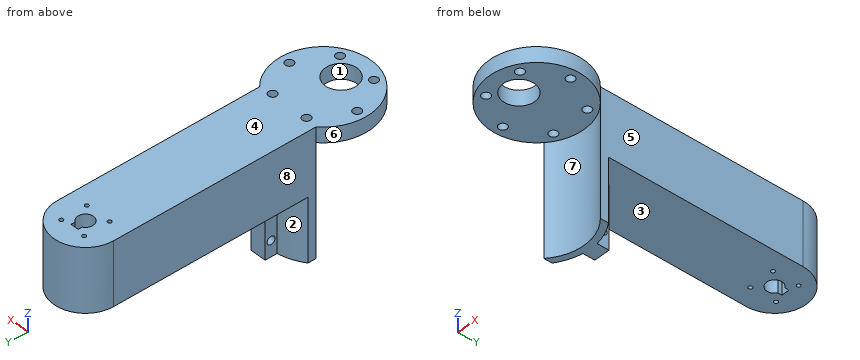
from build123d import *

# Parameters (mm, degrees)
SKETCH1_R           = 3.175
SKETCH1_R_2         = 0.762
BOSS_EXTRUDE1_DEPTH = 25.4
SKETCH2_R           = 19.05
SKETCH2_R_2         = 3.175
BOSS_EXTRUDE2_DEPTH = 25.4
SKETCH3_R           = 1.651
CUT_EXTRUDE1_DEPTH  = 25.4
SKETCH5_R           = 6.35
CUT_EXTRUDE2_DEPTH  = 25.4
SKETCH6_W           = 3.175
SKETCH6_H           = 1.5875
CUT_EXTRUDE3_DEPTH  = 25.4
SKETCH2_2_R         = 3.175
CUT_EXTRUDE6_DEPTH  = 25.4
SKETCH8_R           = 1.651
SKETCH8_R_2         = 6.35
CUT_EXTRUDE4_DEPTH  = 19.3
BOSS_EXTRUDE3_DEPTH = 25.4
SKETCH10_W          = 6.35
SKETCH10_H          = 4.7625
BOSS_EXTRUDE4_DEPTH = 25.4
SKETCH11_R          = 1.5875
CUT_EXTRUDE5_DEPTH  = 23.225


with BuildPart() as part:
    # Sketch1 → Boss-Extrude1 (new body)
    with BuildSketch(Plane.XY):
        with BuildLine():
            Line((12.7, 50.8), (12.7, -50.8))
            ThreePointArc((12.7, -50.8), (0, -63.5), (-12.7, -50.8))
            Line((-12.7, -50.8), (-12.7, 50.8))
            ThreePointArc((-12.7, 50.8), (0, 63.5), (12.7, 50.8))
        make_face()
        with Locations((0, 50.8)):
            Circle(SKETCH1_R, mode=Mode.SUBTRACT)
        with Locations((-5.118745989, 55.918745989)):
            Circle(SKETCH1_R_2, mode=Mode.SUBTRACT)
        with Locations((5.118745989, 55.918745989)):
            Circle(SKETCH1_R_2, mode=Mode.SUBTRACT)
        with Locations((5.118745989, 45.681254011)):
            Circle(SKETCH1_R_2, mode=Mode.SUBTRACT)
        with Locations((-5.118745989, 45.681254011)):
            Circle(SKETCH1_R_2, mode=Mode.SUBTRACT)
    extrude(amount=BOSS_EXTRUDE1_DEPTH)

    # Sketch2 → Boss-Extrude2 (add)
    with BuildSketch(Plane(origin=(0, 0, 0), x_dir=(-1, 0, 0), z_dir=(0, 0, -1))):
        with Locations((0, -44.45)):
            Circle(SKETCH2_R)
        with Locations((0, 50.8)):
            Circle(SKETCH2_R_2)
    extrude(amount=-BOSS_EXTRUDE2_DEPTH)

    # Sketch3 → Cut-Extrude1 (cut)
    with BuildSketch(Plane.XY.offset(25.4)):
        with Locations((-7.62, -30.959275928)):
            Circle(SKETCH3_R)
        with Locations((7.62, -30.959275928)):
            Circle(SKETCH3_R)
        with Locations((-15.24, -44.45)):
            Circle(SKETCH3_R)
        with Locations((-7.62, -57.940724072)):
            Circle(SKETCH3_R)
        with Locations((7.62, -57.940724072)):
            Circle(SKETCH3_R)
        with Locations((15.24, -44.45)):
            Circle(SKETCH3_R)
    extrude(amount=-CUT_EXTRUDE1_DEPTH, mode=Mode.SUBTRACT)

    # Sketch5 → Cut-Extrude2 (cut)
    with BuildSketch(Plane.XY.offset(25.4)):
        with Locations((0, -51.562)):
            Circle(SKETCH5_R)
    extrude(amount=-CUT_EXTRUDE2_DEPTH, mode=Mode.SUBTRACT)

    # Sketch6 → Cut-Extrude3 (cut)
    with BuildSketch(Plane(origin=(0, 0, 0), x_dir=(-1, 0, 0), z_dir=(0, 0, -1))):
        with Locations((0, 54.343380657)):
            Rectangle(SKETCH6_W, SKETCH6_H)
    extrude(amount=-CUT_EXTRUDE3_DEPTH, mode=Mode.SUBTRACT)

    # Sketch2<2> → Cut-Extrude6 (cut)
    with BuildSketch(Plane(origin=(0, 0, 0), x_dir=(-1, 0, 0), z_dir=(0, 0, -1))):
        with Locations((0, 50.8)):
            Circle(SKETCH2_2_R)
    extrude(amount=-CUT_EXTRUDE6_DEPTH, mode=Mode.SUBTRACT)

    # Sketch8 → Cut-Extrude4 (cut)
    with BuildSketch(Plane(origin=(0, 0, 0), x_dir=(-1, 0, 0), z_dir=(0, 0, -1))):
        with BuildLine():
            ThreePointArc((-12.7, -30.250968343), (-7.777129933, -61.840191201), (19.05, -44.45))
            ThreePointArc((19.05, -44.45), (17.390191201, -36.672870067), (12.7, -30.250968343))
            ThreePointArc((12.7, -30.250968343), (0, -25.4), (-12.7, -30.250968343))
        make_face()
        with Locations((-7.62, -57.940724072)):
            Circle(SKETCH8_R, mode=Mode.SUBTRACT)
        with Locations((7.62, -57.940724072)):
            Circle(SKETCH8_R, mode=Mode.SUBTRACT)
        with Locations((0, -51.562)):
            Circle(SKETCH8_R_2, mode=Mode.SUBTRACT)
        with Locations((-15.24, -44.45)):
            Circle(SKETCH8_R, mode=Mode.SUBTRACT)
        with Locations((-7.62, -30.959275928)):
            Circle(SKETCH8_R, mode=Mode.SUBTRACT)
        with Locations((15.24, -44.45)):
            Circle(SKETCH8_R, mode=Mode.SUBTRACT)
        with Locations((7.62, -30.959275928)):
            Circle(SKETCH8_R, mode=Mode.SUBTRACT)
        with Locations((7.62, -30.959275928)):
            Circle(SKETCH8_R)
        with Locations((-7.62, -30.959275928)):
            Circle(SKETCH8_R)
        with Locations((-15.24, -44.45)):
            Circle(SKETCH8_R)
        with Locations((-7.62, -57.940724072)):
            Circle(SKETCH8_R)
        with Locations((0, -51.562)):
            Circle(SKETCH8_R_2)
        with Locations((7.62, -57.940724072)):
            Circle(SKETCH8_R)
        with Locations((15.24, -44.45)):
            Circle(SKETCH8_R)
    extrude(amount=-CUT_EXTRUDE4_DEPTH, mode=Mode.SUBTRACT)

    # Sketch9 → Boss-Extrude3 (add)
    with BuildSketch(Plane(origin=(0, 0, 0), x_dir=(-1, 0, 0), z_dir=(0, 0, -1))):
        with BuildLine():
            Line((-12.7, -30.250968343), (-12.7, -26.990386602))
            ThreePointArc((-12.7, -26.990386602), (0, -22.86), (12.7, -26.990386602))
            Line((12.7, -26.990386602), (12.7, -30.250968343))
            ThreePointArc((12.7, -30.250968343), (0, -25.4), (-12.7, -30.250968343))
        make_face()
    extrude(amount=BOSS_EXTRUDE3_DEPTH)

    # Sketch10 → Boss-Extrude4 (add)
    with BuildSketch(Plane(origin=(0, 0, 0), x_dir=(-1, 0, 0), z_dir=(0, 0, -1))):
        with Locations((0, -20.713481915)):
            Rectangle(SKETCH10_W, SKETCH10_H)
    extrude(amount=BOSS_EXTRUDE4_DEPTH)

    # Sketch11 → Cut-Extrude5 (cut, through all)
    with BuildSketch(Plane(origin=(3.175, 0, 0), x_dir=(0, 0, -1), z_dir=(1, 0, 0))):
        with Locations((6.35, -20.713481915)):
            Circle(SKETCH11_R)
        with Locations((19.05, -20.713481915)):
            Circle(SKETCH11_R)
    extrude(amount=-CUT_EXTRUDE5_DEPTH, mode=Mode.SUBTRACT)


solid = part.part
The model under review builds one solid part; all positions refer to its coordinate system, in mm. Face numbers are marked on the shaded views. A direction names the side the tool comes from. Coordinates: 2 decimals unless noted, no trailing zeros. Order: outer loops, then holes, each group sorted by start corner. A loop starts at its lowest first (then second) coordinate and runs counter-clockwise, first axis right, second up. Notation, with made-up numbers: (-23, 87.5) -> (-5, 87.5) arc R14 ccw to (-5, 91.5) -> close; hole circle Ø11 at (-20, 30.25). An arc over 180 degrees is marked (long way). Answer in a Markdown table with one row per item.
(1) Consider section C-C (z = -12.5). Write out the cut boundary in (x, y) (3 decimals), plus the area to 3 significant figures.
Answers:
| item | result |
|---|---|
| outline | (-12.7, -30.251) arc R19.05 cw to (12.7, -30.251) -> (12.7, -26.99) arc R21.59 ccw to (3.175, -23.095) -> (3.175, -18.332) -> (-3.175, -18.332) -> (-3.175, -23.095) arc R21.59 ccw to (-12.7, -26.99) -> close |
| area | 99.0 mm² |
(2) Wall thickness on line 1 along Y through (x, z) = (1, -19); line 2 along Y through (x, z) = (7.62, 20.5); line 3 along Y through (x, z) = (-2.5, 23): over which ranges is each line inside the solid? List them lowest first.
Answers:
| item | result |
|---|---|
| line 1 | -25.43 to -22.3, -19.13 to -18.33 |
| line 2 | -61.91 to -59.59, -56.29 to -32.61, -29.31 to 60.96 |
| line 3 | -63.34 to -57.4, -45.72 to 48.84, 52.76 to 63.25 |
(3) Consider section B-B (x = -7.62). Write out the cut boundary in (y, z), plus the area to 3 significant figures.
Answers:
| item | result |
|---|---|
| outline | (-61.91, 19.3) -> (-59.59, 19.3) -> (-59.59, 25.4) -> (-61.91, 25.4) -> close; (-56.29, 19.3) -> (-32.61, 19.3) -> (-32.61, 25.4) -> (-56.29, 25.4) -> close; (-29.31, 19.3) -> (-26.99, 19.3) -> (-26.99, -25.4) -> (-24.25, -25.4) -> (-24.25, 0) -> (60.96, 0) -> (60.96, 25.4) -> (-29.31, 25.4) -> close |
| area | 2,480 mm² |
(4) Machinability: for the marked faces 4, 5, 6, 7 and 8, which of the approach directions +Z, -Z, +X, -X, +Y, -Y give a long, thin tool a straight path to every point of the face, cutting with its end or side? Answer none if there is none.
Answers:
| item | result |
|---|---|
| face 4 | +Z, +X, -X, +Y, -Y |
| face 5 | +Z, -Z, +X, +Y |
| face 6 | +Z, -Z |
| face 7 | -Z, -Y |
| face 8 | +Z, -Z, -X, +Y |
(5) Insertion check: pin 1 (6 mm diameter, centred on x = -2.5, y = 48.5, fed in from -Z); pin 2 (5 mm diameter, centred on y = 3, z = 4.5, fed in from +X); pin 3 (2 mm diameter, centred on x = 7.62, y = -30.96, fed in from -Z); pin 4 (4 mm diameter, centred on y = -20.71, z = -6.35, fed in from -X) (3 decimals). Each pin has a flat end and moves straight along its axis. Give the tip position at first contact, or say it passes through.
Answers:
| item | result |
|---|---|
| pin 1 | z = 0 |
| pin 2 | x = 12.7 |
| pin 3 | through |
| pin 4 | x = -3.175 |
(6) Consider section A-A (x = -15.24). Write out the cut boundary in (y, z), plus the area to 3 significant figures.
Answers:
| item | result |
|---|---|
| outline | (-55.88, 19.3) -> (-46.1, 19.3) -> (-46.1, 25.4) -> (-55.88, 25.4) -> close; (-42.8, 19.3) -> (-33.02, 19.3) -> (-33.02, 25.4) -> (-42.8, 25.4) -> close |
| area | 119 mm² |
(7) The part is to be moulded in two halves that separate along Y. For the marked faces 1, 2 and 3, say which applies: +Y half, -Y half, draft (parallel to the pull), parting line (faces both ways), or undercut.
Answers:
| item | result |
|---|---|
| face 1 | undercut |
| face 2 | +Y half |
| face 3 | draft |
(8) Consider section D-D (x = 0). State how many separate pieces and enclosed holes the cut face has, plus the area to 3 significant figures.
Answers:
| item | result |
|---|---|
| separate pieces | 3 |
| enclosed holes | 2 |
| area | 2,390 mm² |
